CAD build for the part. Positions are in the model's coordinates, mm. Face numbers are marked on the shaded views. A direction names the side the tool comes from. Coordinates: 2 decimals unless noted, no trailing zeros. Order: outer loops, then holes, each group sorted by start corner. A loop starts at its lowest first (then second) coordinate and runs counter-clockwise, first axis right, second up.
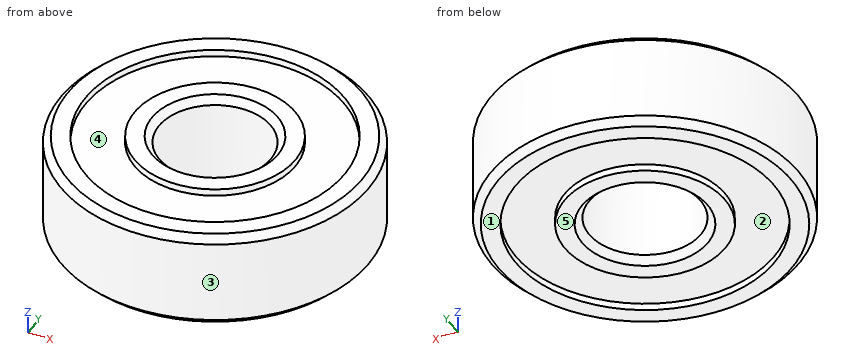
from build123d import *

# Parameters (mm, degrees)
F0_R     = 11
F0_R_2   = 4
F1_DEPTH = 3.5
F2_SIZE  = 0.5
F3_W     = 3.5
F3_H     = 0.5
F3_H_2   = 1


with BuildPart() as f1:
    # F0 (on Top) → F1 (new body, symmetric)
    with BuildSketch(Plane.XY):
        Circle(F0_R)
        Circle(F0_R_2, mode=Mode.SUBTRACT)
    extrude(amount=F1_DEPTH, both=True)

    # F2
    f2_edges = [f1.edges().sort_by_distance(p)[0] for p in [
        (-11, 0, 3.5),
        (-11, 0, -3.5),
        (-4, 0, 3.5),
        (-4, 0, -3.5),
    ]]
    chamfer(f2_edges, length=F2_SIZE)

    # F3 (on Right) → F4 (revolve, cut)
    with BuildSketch(Plane.YZ):
        with Locations((7.5, 3.75)):
            Rectangle(F3_W, F3_H)
        with Locations((7.5, 3.25)):
            Rectangle(F3_W, F3_H)
        with Locations((7.5, -3.5)):
            Rectangle(F3_W, F3_H_2)
    revolve(axis=Axis((0, 0, 3.5), (0, 0, 1)), mode=Mode.SUBTRACT)


solid = f1.part
1) Two-plate mould, pull along Y, no slides. Class the marked faces 3, 4 and 5: released by +Y, released by -Y, zero draft, split by the parting line, or undercut.
2) Which spindle directions (+Z, -Z, +X, -X, +Y, -Y) get a long thin tool onto all of the face, cutting with end or side? Do the marked faces 1 and 2. Say none if no direction does.
3) Pin check, flat tips, straight feed: P1, Ø4, axis at x = -3, z = 2.5, coming from the -Y side; P2, Ø1.5, axis at y = 3.5, z = 0.5, coming from the +X side; P3, Ø1, axis at x = -1.5, z = 1, coming from the +Y side; P4, Ø2, axis at x = 2.5, y = 1.5, coming from the +Z side. Stop position of each tip, or through.
4) Slice it at C-C (z = 2.25). List the corners of the cut face in (x, y), plus the area to 3 significant figures.
5) Drill centre lines: probe 1 along Y at (x, z) = (0, 3.35); probe 2 along X at (y, z) = (0, -3.25); probe 3 along Y at (x, z) = (0, -3.15). Where is each one in solid material? Low to high.
Worked out:
1. face 3: split by the parting line
1. face 4: undercut
1. face 5: zero draft
2. face 1: -Z, +X, -X, +Y, -Y
2. face 2: -Z
3. P1: stops at y = -10.95
3. P2: stops at x = 10.65
3. P3: stops at y = 10.95
3. P4: passes through
4. outline: circle Ø22 at (0, 0); hole circle Ø8 at (0, 0)
4. area: 330 mm2
5. probe 1: y = -10.65 to -9.25, -5.75 to -4.35, 4.35 to 5.75, 9.25 to 10.65
5. probe 2: x = -10.75 to -9.25, -5.75 to -4.25, 4.25 to 5.75, 9.25 to 10.75
5. probe 3: y = -10.85 to -9.25, -5.75 to -4.15, 4.15 to 5.75, 9.25 to 10.85
